Part model, mm, in its own coordinate system. Give positions to 0.01 mm unless a question says otherwise; leave off trailing zeros. Loops run counter-clockwise (first coordinate to the right, second up) from the corner with the lowest first, then second, coordinate; pieces in that order, holes last. Notation, with made-up numbers: M 4,70.25 L 53,70.25 A9 ccw 53,80.25 Z; hole C -34.5,-30 d10. An arc over 180 degrees is marked long. Answer in a Markdown table with one row per item.
from build123d import *

# Parameters (mm, degrees)
F0_W     = 165
F0_H     = 85
F0_R     = 2.1
F0_R_2   = 12.5
F0_R_3   = 9.525
F1_DEPTH = 3.175
F2_R     = 1.778
F3_DEPTH = 3.175


with BuildPart() as f1:
    # F0 (on Top) → F1 (new body)
    with BuildSketch(Plane.XY):
        with Locations((31.925802, 2.240353)):
            Rectangle(F0_W, F0_H)
        with Locations((-5.574198, -22.759647)):
            Circle(F0_R, mode=Mode.SUBTRACT)
        with Locations((-30.574198, 2.240353)):
            Circle(F0_R, mode=Mode.SUBTRACT)
        with Locations((-5.574198, 2.240353)):
            Circle(F0_R_2, mode=Mode.SUBTRACT)
        with Locations((19.425802, 2.240353)):
            Circle(F0_R, mode=Mode.SUBTRACT)
        with Locations((-5.574198, 27.240353)):
            Circle(F0_R, mode=Mode.SUBTRACT)
        with Locations((69.425802, 2.240353)):
            Circle(F0_R_3, mode=Mode.SUBTRACT)
    extrude(amount=F1_DEPTH)

    # F2 (on face) → F3 (cut, through all)
    with BuildSketch(Plane.XY.offset(3.175)):
        with Locations((-44.224198, 38.390353)):
            Circle(F2_R)
        with Locations((-44.224198, -33.909647)):
            Circle(F2_R)
        with Locations((108.075802, 38.390353)):
            Circle(F2_R)
        with Locations((108.075802, -33.909647)):
            Circle(F2_R)
    extrude(amount=-F3_DEPTH, mode=Mode.SUBTRACT)


solid = f1.part
(1) Pin check, flat tips, straight feed: pin 1 Ø5.5 at (x, y) = (-5.57, -22.76) entering from +Z (3 decimals); pin 2 Ø3 at (x, y) = (-44.22, 38.39) entering from +Z. Stop position of each tip, or through.
Recorded:
| item | result |
|---|---|
| pin 1 | stops at z = 3.175 |
| pin 2 | passes through |
(2) Saw through at B-B (y = 10). Write the cut outline in (x, z) (3 decimals), plus the area to 3 significant figures.
Recorded:
| item | result |
|---|---|
| outline | M -50.574,0 L -15.374,0 L -15.374,3.175 L -50.574,3.175 Z; M 4.226,0 L 63.902,0 L 63.902,3.175 L 4.226,3.175 Z; M 74.95,0 L 114.426,0 L 114.426,3.175 L 74.95,3.175 Z |
| area | 427 mm^2 |
(3) Saw through at D-D (y = -4.5). Write the cut outline in (x, z) (3 decimals).
Recorded:
| item | result |
|---|---|
| outline | M -50.574,0 L -16.101,0 L -16.101,3.175 L -50.574,3.175 Z; M 4.953,0 L 62.696,0 L 62.696,3.175 L 4.953,3.175 Z; M 76.156,0 L 114.426,0 L 114.426,3.175 L 76.156,3.175 Z |
(4) Saw through at C-C (z = 0.65). Give the number of separate pieces and of enclosed holes in the cut face, plus the area to 3 significant figures.
Recorded:
| item | result |
|---|---|
| separate pieces | 1 |
| enclosed holes | 10 |
| area | 13,200 mm^2 |
(5) Pull direction Y, two halves, no side cores. Call faces 1 (the face through (31, -40.26, 2)), 2 (the face through (-45.535, -32.708, 1.61)), 3 (the face through (114.426, 2, 2)): +Y half, -Y half, draft (parallel to the pull), parting line (faces both ways), or undercut.
Recorded:
| item | result |
|---|---|
| face 1 | -Y half |
| face 2 | undercut |
| face 3 | draft |
(6) Drill centre lines: line 1 along Y through (x, z) = (-5, 2.85); line 2 along X through (y, z) = (9, 2.65); line 3 along X through (y, z) = (-4, 1.8). Where is each one in solid material? Low to high.
Recorded:
| item | result |
|---|---|
| line 1 | y = -40.26 to -24.78, -20.74 to -10.25, 14.73 to 25.22, 29.26 to 44.74 |
| line 2 | x = -50.57 to -16.09, 4.94 to 62.72, 76.14 to 114.43 |
| line 3 | x = -50.57 to -16.41, 5.26 to 62.23, 76.62 to 114.43 |
(7) Saw through at A-A (x = 64). Write the cut outline in (y, z) (3 decimals).
Recorded:
| item | result |
|---|---|
| outline | M -40.26,0 L -5.588,0 L -5.588,3.175 L -40.26,3.175 Z; M 10.069,0 L 44.74,0 L 44.74,3.175 L 10.069,3.175 Z |
